Geometry: final body of the model. Coordinates: model frame, mm. Face numbers are marked on the shaded views. A direction names the side the tool comes from. Coordinates: 2 decimals unless noted, no trailing zeros. Order: outer loops, then holes, each group sorted by start corner. A loop starts at its lowest first (then second) coordinate and runs counter-clockwise, first axis right, second up. Notation, with made-up numbers: M 1.5,66.25 L 44.5,66.25 A20 cw 44.5,91.25 Z; hole C -4.75,4 d2. An arc over 180 degrees is marked long. Use CSV: the item, a comma, the result in double quotes. Start each with the question number.
Q1. Mould query, pull axis X, two halves, no side actions, for the marked faces 1, 2 and 3. Classes: +X half, -X half, draft (parallel to the pull), parting line (faces both ways), or undercut.
Q2. Section query C-C, the plane z = 61. Output: boundary loops of the cut face in (x, y).
Q3. Section query A-A, the plane z = 95. Output: boundary loops of the cut face in (x, y), and give its area (3 significant figures).
Q4. Section query D-D, the plane y = 99. Output: boundary loops of the cut face in (x, z).
Q5. First-contact query: P1, Ø6, axis at x = 21.5, y = 38, coming from the +Z side; P2, Ø3, axis at x = 20.5, y = 33.5, coming from the -Z side; P3, Ø4, axis at y = 32.5, z = 95, coming from the -X side. Flat tips, straight axial feed; report the tip coordinate or a pass-through.
Q6. Ray query, probe 1 along Y at (x, z) = (10, 41); probe 2 along Z at (x, y) = (90.5, 34.5); probe 3 along Z at (x, y) = (12, 60). Return the intervals inside material, ascending.
Q7. Access query for the marked faces 4, 5 and 6. Directions: +Z, -Z, +X, -X, +Y, -Y. A direction counts if a zero-diameter tool reaches every point of the face in a straight line with its end or side. Return the directions, or none.
Q8. Section query B-B, the plane x = -21. Output: boundary loops of the cut face in (y, z), and give its area (3 significant figures).
from build123d import *

# Parameters (mm, degrees)
MAIN_BUILDING_DEPTH       = 80
SMALL_BUILDING_DEPTH      = 35
SMALL_BUILDING_ROOF_DEPTH = 70


with BuildPart() as part:
    # Sketch1 → Main Building (new body)
    with BuildSketch(Plane(origin=(0, 0, 0), x_dir=(1, 0, 0), z_dir=(0, 1, 0))):
        Polygon((0, 0), (-65, -112.583302492), (-13.038475773, -142.583302492), (51.961524227, -30), align=None)
    extrude(amount=MAIN_BUILDING_DEPTH)

    # Sketch2 → Dome (revolve)
    with BuildSketch(Plane(origin=(0, 80, 0), x_dir=(-1, 0, 0), z_dir=(0, 1, 0))):
        with BuildLine():
            Line((24.019237886, 71.602540378), (24.019237886, 131.602540378))
            ThreePointArc((24.019237886, 131.602540378), (-5.980762114, 101.602540378), (24.019237886, 71.602540378))
        make_face()
    revolve(axis=Axis((-24.019237886, 80, 71.602540378), (0, 0, 1)))

    # Sketch3 → Small Building (add)
    with BuildSketch(Plane(origin=(0, 0, 0), x_dir=(1, 0, 0), z_dir=(0, 1, 0))):
        Polygon((51.961524227, -30), (112.583302492, -65), (87.583302492, -108.301270189), (26.961524227, -73.301270189), align=None)
    extrude(amount=SMALL_BUILDING_DEPTH)

    # Sketch4 → Small Building Roof (add)
    with BuildSketch(Plane(origin=(112.583302492, 0, 65), x_dir=(0.5, 0, -0.866025404), z_dir=(0.866025404, 0, 0.5))):
        Polygon((0, 35), (-50, 35), (-25, 50), align=None)
    extrude(amount=-SMALL_BUILDING_ROOF_DEPTH)


solid = part.part
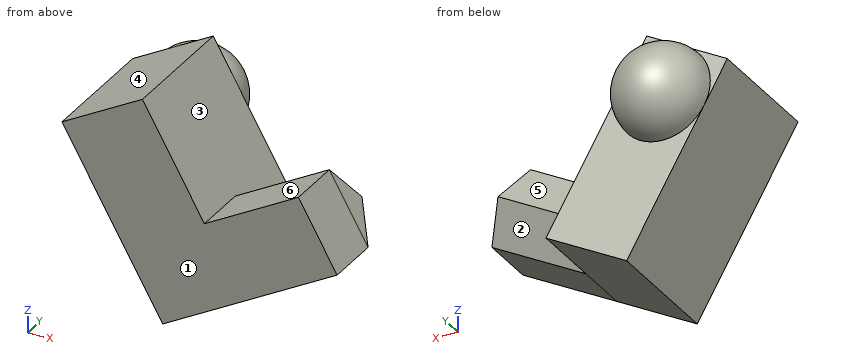
Responses:
1,face 1,"draft"
1,face 2,"+X half"
1,face 3,"undercut"
2,outline,"M -35.22,0 L 105.66,0 L 105.66,35 L 55.66,50 L 34.06,43.52 L 34.06,80 L -35.22,80 Z"
3,outline,"M -54.85,0 L 14.43,0 L 14.43,80 L 5.25,80 A29.26 ccw -53.28,80 L -54.85,80 Z; M 64.54,0 L 95.26,0 L 95.26,44.22 L 64.54,35 Z"
3,area,"8,100 mm²"
4,outline,"C -24.02,101.6 d46.43"
5,P1,"stops at z = 87.96"
5,P2,"stops at z = 10.97"
5,P3,"stops at x = -56"
6,probe 1,"y = 0 to 80"
6,probe 2,"z = 52.25 to 103.25"
6,probe 3,"z = 6.93 to 99.22"
7,face 4,"+Z, -X, +Y, -Y"
7,face 5,"+Z, +Y"
7,face 6,"+Z, +Y, -Y"
8,outline,"M 0,36.37 L 80,36.37 L 80,71.75 A29.85 ccw 80,131.45 L 80,137.99 L 0,137.99 Z"
8,area,"9,530 mm²"
